Design review of the part built by this model. Coordinates are the model's own, in mm. A direction names the side the tool comes from. Coordinates: 2 decimals unless noted, no trailing zeros. Answer in a Markdown table with one row per item. Add a question column.
Item 1: Draft analysis for pull direction Z (two halves, no side actions). For faces 1 (the face through (13.057, 2, 1)), 2 (the face through (6.132, 2, 6)), state which applies: released by +Z, released by -Z, zero draft, split by the parting line, or undercut.
Item 2: To check wall thickness, follow line 1 (Z direction, x = 13, y = 1.65); line 2 (Z direction, x = 22.5, y = 0.5); line 3 (X direction, y = 2.7, z = -9). State the ranges of each line that lie inside material, in increasing order.
Item 3: Take a section at A-A, the plane y = 2.4. Give the number of separate pieces and of enclosed holes in the cut face, and give its area (3 significant figures).
Item 4: For faces 3 (the face through (6.132, 2, -5)), 4 (the face through (10, 2, -0.028)), list the 3-axis set-ups (+Z, -Z, +X, -X, +Y, -Y) from which the entire face can be reached by the end or side of a thin tool; tool diameter is ignored.
from build123d import *

# Parameters (mm, degrees)
SKETCH1_W           = 50.8
SKETCH1_H           = 21.59
BOSS_EXTRUDE1_DEPTH = 3.175
FILLET1_R           = 10.16
SKETCH3_R           = 1.16713
CUT_EXTRUDE1_DEPTH  = 28.780796425
FILLET3_R           = 10.16
SCALE1_SCALE_X      = 1.3
SCALE1_SCALE_Y      = 1
SCALE1_SCALE_Z      = 1.3
SKETCH4_W           = 39.116
SKETCH4_H           = 28.067
CUT_EXTRUDE2_DEPTH  = 37.054605389
FILLET4_R           = 3.175
SKETCH7_W           = 6.925112
SKETCH7_H           = 1.2
CUT_EXTRUDE3_DEPTH  = 37.054605389


with BuildPart() as part:
    # Sketch1 → Boss-Extrude1 (new body)
    with BuildSketch(Plane(origin=(0, 0, 0), x_dir=(1, 0, 0), z_dir=(0, 1, 0))):
        Rectangle(SKETCH1_W, SKETCH1_H)
    extrude(amount=BOSS_EXTRUDE1_DEPTH)

    # Fillet1
    fillet1_edges = [part.edges().sort_by_distance(p)[0] for p in [
        (25.4, 1.5875, 10.795),
        (-25.4, 1.5875, 10.795),
    ]]
    fillet(fillet1_edges, radius=FILLET1_R)

    # Sketch3 → Cut-Extrude1 (cut, through all)
    with BuildSketch(Plane(origin=(0, 3.175, 0), x_dir=(1, 0, 0), z_dir=(0, 1, 0))):
        with Locations(Location((15.24, -0.635, 0), (0, 0, 270))):
            Circle(SKETCH3_R)
        with Locations(Location((16.637, 6.855847148, 0), (0, 0, 270))):
            Circle(SKETCH3_R)
        with Locations(Location((-3.81, -0.635, 0), (0, 0, 270))):
            Circle(SKETCH3_R)
    extrude(amount=-CUT_EXTRUDE1_DEPTH, mode=Mode.SUBTRACT)

    # Fillet3
    fillet3_edges = [part.edges().sort_by_distance(p)[0] for p in [
        (-25.4, 1.5875, -10.795),
        (25.4, 1.5875, -10.795),
    ]]
    fillet(fillet3_edges, radius=FILLET3_R)


with BuildPart() as part_1:
    # Scale1: scaled about (-0.120675705, 1.5875, 0.024016676)
    add(part.part.scale((SCALE1_SCALE_X, SCALE1_SCALE_Y, SCALE1_SCALE_Z), about=(-0.120675705, 1.5875, 0.024016676)))

    # Sketch4 → Cut-Extrude2 (cut, through all)
    with BuildSketch(Plane(origin=(0, 3.175, 0), x_dir=(1, 0, 0), z_dir=(0, 1, 0))):
        with Locations((-13.425797288, 0.007205003)):
            Rectangle(SKETCH4_W, SKETCH4_H)
    extrude(amount=-CUT_EXTRUDE2_DEPTH, mode=Mode.SUBTRACT)

    # Fillet4
    fillet4_edges = [part_1.edges().sort_by_distance(p)[0] for p in [
        (6.132202712, 1.5875, -14.040705003),
        (6.132202712, 1.5875, 14.026294997),
    ]]
    fillet(fillet4_edges, radius=FILLET4_R)

    # Sketch7 → Cut-Extrude3 (cut, through all)
    with BuildSketch(Plane.XZ):
        with Locations((9.594758712, 0.571779506)):
            Rectangle(SKETCH7_W, SKETCH7_H)
    extrude(amount=-CUT_EXTRUDE3_DEPTH, mode=Mode.SUBTRACT)


solid = part_1.part
Answers:
| question | item | result |
|---|---|---|
| 1 | face 1 | undercut |
| 1 | face 2 | zero draft |
| 2 | line 1 | z = -14.04 to -0.03, 1.17 to 14.03 |
| 2 | line 2 | z = -13.77 to -10.19, -7.65 to 13.76 |
| 2 | line 3 | x = 6.13 to 20.15, 23.18 to 30.23 |
| 3 | separate pieces | 1 |
| 3 | enclosed holes | 2 |
| 3 | area | 654 mm^2 |
| 4 | face 3 | +Z, -Z, -X, +Y, -Y |
| 4 | face 4 | -X, +Y, -Y |
